Here's how the part is built. I have some questions about the finished solid (model axes, mm). A direction names the side the tool comes from. Round coordinates to 2 decimals unless told otherwise and drop trailing zeros. Write each loop counter-clockwise with the first axis right and the second up, starting at its lowest first coordinate (ties: lowest second). Pieces come first, ordered by that corner, then holes. Notation, with made-up numbers: M 45.5,-1 L 56.5,-1 A18 ccw 56.5,34 Z; hole C 56,41 d1. An arc over 180 degrees is marked long. Use one line per item in the form item = value. Start each with the question number.
Q1. I need wall thicknesses on line 1 along X through (y, z) = (1, -3.5); line 2 along Z through (x, y) = (42, 8.5); line 3 along X through (y, z) = (0.75, -3.75). Which ranges of each line are inside material? Lowest first, please. Write a range as from..to.
Q2. We'd pull the mould along Z, two halves only. Please class faces 1 (the face through (-20.305, 7.479, -6.342)), 2 (the face through (9.237, 1.479, -6.469)), 3 (the face through (17.695, 1.479, 5.031)), 4 (the face through (26.7, 1.5, -3.7)): +Z half, -Z half, draft (parallel to the pull), parting line (faces both ways), or undercut.
Q3. I want a section at C-C on x = 18. List the corners of the cut face in (y, z) for me, and give its area (3 significant figures).
Q4. For faces 5 (the face through (44, 3, -2.24)), 6 (the face through (19.216, 1, 2)), 7 (the face through (-5.756, 4.972, -3.427)), 8 (the face through (-12.534, 1.014, -1.028)), which set-ups out of +Z, -Z, +X, -X, +Y, -Y let a thin tool reach every point of the face, with its end or its side?
Q5. I want a section at B-B on y = 4.5. State how many separate pieces and enclosed holes the cut face has, and give its area (3 significant figures).
Q6. I want a section at A-A on x = 37.5. List the corners of the cut face in (y, z) for me.
Q7. I'm going to push flat-ended pins straight in: pin 1 Ø6 at (x, z) = (4.5, 4) entering from +Y; pin 2 Ø3.5 at (x, y) = (-18.28, 4.5) entering from +Z; pin 3 Ø1.5 at (x, y) = (12, 2) entering from -Z. Where does each tip first touch, or does it pass through?
```python
from build123d import *

# Parameters (mm, degrees)
BOSS_EXTRU_1_DEPTH      = 3
ESQUISSE2_W             = 14
ESQUISSE2_H             = 9
BOSS_EXTRU_2_DEPTH      = 6
ESQUISSE3_R             = 3.25
ENL_V_MAT_EXTRU_1_DEPTH = 50.69554375
CHANFREIN1_SIZE         = 4
ESQUISSE4_R             = 1.5
ENL_V_MAT_EXTRU_2_DEPTH = 50.240705403
ESQUISSE5_W             = 9.5
ESQUISSE5_H             = 2.5
ENL_V_MAT_EXTRU_3_DEPTH = 50.69554375
ESQUISSE6_R             = 1.5
ENL_V_MAT_EXTRU_4_DEPTH = 50.86789407
CHANFREIN2_SIZE         = 3
CHANFREIN3_SIZE         = 3
BOSS_EXTRU_3_START      = -2
BOSS_EXTRU_3_DEPTH      = 2


with BuildPart() as part:
    # Esquisse1 → Boss.-Extru.1 (new body)
    with BuildSketch(Plane(origin=(0, 0, 0), x_dir=(1, 0, 0), z_dir=(0, 1, 0))):
        Polygon((-21.783749016, 7.99000686), (10.716250984, 7.99000686), (10.716250984, 2.552277958), (15.716250984, 2.552277958), (15.716250984, 7.99000686), (48.216250984, 7.99000686), (48.216250984, -1.00999314), (19.216250984, -1.00999314), (19.216250984, -6.50999314), (7.216250984, -6.50999314), (7.216250984, -1.00999314), (-21.783749016, -1.00999314), align=None)
    extrude(amount=BOSS_EXTRU_1_DEPTH)

    # Esquisse2 → Boss.-Extru.2 (add)
    with BuildSketch(Plane(origin=(0, 3, 0), x_dir=(1, 0, 0), z_dir=(0, 1, 0))):
        with Locations((-14.783749016, 3.49000686)):
            Rectangle(ESQUISSE2_W, ESQUISSE2_H)
        with Locations((41.216250984, 3.49000686)):
            Rectangle(ESQUISSE2_W, ESQUISSE2_H)
    extrude(amount=BOSS_EXTRU_2_DEPTH)

    # Esquisse3 → Enlèv. mat.-Extru.1 (cut, through all)
    with BuildSketch(Plane(origin=(0, 9, 0), x_dir=(1, 0, 0), z_dir=(0, 1, 0))):
        with Locations(Location((-12.283749016, 3.49000686, 0), (0, 0, 270))):
            Circle(ESQUISSE3_R)
        with Locations(Location((38.716250984, 3.49000686, 0), (0, 0, 270))):
            Circle(ESQUISSE3_R)
    extrude(amount=-ENL_V_MAT_EXTRU_1_DEPTH, mode=Mode.SUBTRACT)

    # Chanfrein1
    chanfrein1_edges = [part.edges().sort_by_distance(p)[0] for p in [
        (-7.783749016, 3, -3.49000686),
        (34.216250984, 3, -3.49000686),
    ]]
    chamfer(chanfrein1_edges, length=CHANFREIN1_SIZE)

    # Esquisse4 → Enlèv. mat.-Extru.2 (cut, through all)
    with BuildSketch(Plane(origin=(0, 3, 0), x_dir=(1, 0, 0), z_dir=(0, 1, 0))):
        with Locations(Location((1.216250984, 3.49000686, 0), (0, 0, 270))):
            Circle(ESQUISSE4_R)
        with Locations(Location((25.216250984, 3.49000686, 0), (0, 0, 270))):
            Circle(ESQUISSE4_R)
        with Locations(Location((13.216250984, -3.50999314, 0), (0, 0, 270))):
            Circle(ESQUISSE4_R)
    extrude(amount=-ENL_V_MAT_EXTRU_2_DEPTH, mode=Mode.SUBTRACT)

    # Esquisse5 → Enlèv. mat.-Extru.3 (cut, through all)
    with BuildSketch(Plane(origin=(0, 9, 0), x_dir=(1, 0, 0), z_dir=(0, 1, 0))):
        with Locations((-17.033749016, 3.49000686)):
            Rectangle(ESQUISSE5_W, ESQUISSE5_H)
        with Locations((43.466250984, 3.49000686)):
            Rectangle(ESQUISSE5_W, ESQUISSE5_H)
    extrude(amount=-ENL_V_MAT_EXTRU_3_DEPTH, mode=Mode.SUBTRACT)

    # Esquisse6 → Enlèv. mat.-Extru.4 (cut, through all)
    with BuildSketch(Plane.XY.offset(1.00999314)):
        with Locations((-18.283749016, 4.5)):
            Circle(ESQUISSE6_R)
        with Locations((44.716250984, 4.5)):
            Circle(ESQUISSE6_R)
    extrude(amount=-ENL_V_MAT_EXTRU_4_DEPTH, mode=Mode.SUBTRACT)

    # Chanfrein2
    chanfrein2_edges = [part.edges().sort_by_distance(p)[0] for p in [
        (48.216250984, 9, -6.36500686),
        (-21.783749016, 9, -6.36500686),
        (48.216250984, 9, -0.61500686),
        (-21.783749016, 9, -0.61500686),
    ]]
    chamfer(chanfrein2_edges, length=CHANFREIN2_SIZE)

    # Chanfrein3
    chanfrein3_edges = [part.edges().sort_by_distance(p)[0] for p in [
        (19.216250984, 1.5, 6.50999314),
        (7.216250984, 1.5, 6.50999314),
        (15.716250984, 1.5, -7.99000686),
        (10.716250984, 1.5, -7.99000686),
    ]]
    chamfer(chanfrein3_edges, length=CHANFREIN3_SIZE)

    # Esquisse7 → Boss.-Extru.3 (add)
    with BuildSketch(Plane.XZ.offset(BOSS_EXTRU_3_START)):
        with BuildLine():
            Line((-10.399834705, -1.885766111), (-9.033749016, -3.49000686))
            ThreePointArc((-9.033749016, -3.49000686), (-11.646371576, -0.303119664), (-15.283749016, -2.24000686))
            Line((-15.283749016, -2.24000686), (-14.419216531, -2.24000686))
            ThreePointArc((-14.419216531, -2.24000686), (-12.500984788, -1.025147811), (-10.399834705, -1.885766111))
        make_face()
        with BuildLine():
            Line((-14.419216531, -4.74000686), (-15.283749016, -4.74000686))
            ThreePointArc((-15.283749016, -4.74000686), (-11.646371576, -6.676894056), (-9.033749016, -3.49000686))
            Line((-9.033749016, -3.49000686), (-10.399834705, -5.094247608))
            ThreePointArc((-10.399834705, -5.094247608), (-12.500984788, -5.954865908), (-14.419216531, -4.74000686))
        make_face()
        with BuildLine():
            ThreePointArc((41.716250984, -2.24000686), (38.078873545, -0.303119664), (35.466250984, -3.49000686))
            Line((35.466250984, -3.49000686), (36.832336674, -1.885766111))
            ThreePointArc((36.832336674, -1.885766111), (38.933486757, -1.025147811), (40.8517185, -2.24000686))
            Line((40.8517185, -2.24000686), (41.716250984, -2.24000686))
        make_face()
        with BuildLine():
            Line((36.832336674, -5.094247608), (35.466250984, -3.49000686))
            ThreePointArc((35.466250984, -3.49000686), (38.078873545, -6.676894056), (41.716250984, -4.74000686))
            Line((41.716250984, -4.74000686), (40.8517185, -4.74000686))
            ThreePointArc((40.8517185, -4.74000686), (38.933486757, -5.954865908), (36.832336674, -5.094247608))
        make_face()
    extrude(amount=BOSS_EXTRU_3_DEPTH)


solid = part.part
```
Reported:
q1.line_1 = -9.04..-0.28, 2.72..10.72, 15.72..23.72, 26.72..35.47
q1.line_2 = -7.99..-4.74, -2.24..1.01
q1.line_3 = -9.26..-0.26, 2.69..10.72, 15.72..23.74, 26.69..35.69
q2.face_1 = draft
q2.face_2 = -Z half
q2.face_3 = +Z half
q2.face_4 = undercut
q3.outline = M 0,-7.27 L 3,-7.27 L 3,4.73 L 0,4.73 Z
q3.area = 36.0 mm^2
q4.face_5 = +X, +Y, -Y
q4.face_6 = +Z, +X, +Y, -Y
q4.face_7 = +Z, -Z, +Y
q4.face_8 = +Y, -Y
q5.separate_pieces = 6
q5.enclosed_holes = 0
q5.area = 160 mm^2
q6.outline = M 0,-7.99 L 9,-7.99 L 9,-6.5 L 2,-6.5 L 2,-5.64 L 0,-5.64 Z; M 0,-1.34 L 2,-1.34 L 2,-0.48 L 9,-0.48 L 9,1.01 L 0,1.01 Z
q7.pin_1 = 3
q7.pin_2 = 1.01
q7.pin_3 = -2.55
